```python
from build123d import *

# Parameters (mm, degrees)
SKETCH1_R                 = 20
BOSS_EXTRUDE1_DEPTH       = 25
BOSS_EXTRUDE2_START       = 100
SKETCH2_R                 = 20
BOSS_EXTRUDE2_DEPTH       = 100
BOSS_EXTRUDE4_START       = -100
SKETCH6_R                 = 20
BOSS_EXTRUDE4_DEPTH       = 100
SKETCH7_R                 = 25
CUT_EXTRUDE2_DEPTH        = 40
SKETCH8_R                 = 25
SKETCH8_R_2               = 22.5
BOSS_EXTRUDE7_DEPTH       = 40
SKETCH9_R                 = 25
BOSS_EXTRUDE8_DEPTH       = 2
BOSS_EXTRUDE10_DEPTH      = 38
CUT_EXTRUDE3_DEPTH        = 25
SKETCH12_R                = 25
CUT_EXTRUDE4_DEPTH        = 75
BOSS_EXTRUDE11_START      = 50
SKETCH14_R                = 20
BOSS_EXTRUDE11_DEPTH      = 50
BOSS_EXTRUDE12_DEPTH      = 10
BOSS_EXTRUDE12_DEPTH_BACK = 50
SKETCH13_R                = 37.5
SKETCH17_R                = 32.5
CUT_EXTRUDE5_DEPTH        = 50
BOSS_EXTRUDE13_START      = 2
SKETCH18_R                = 37.5
SKETCH18_R_2              = 32.5
BOSS_EXTRUDE13_DEPTH      = 2
SKETCH21_R                = 37.5
SKETCH21_R_2              = 32.5
CUT_EXTRUDE6_DEPTH        = 2
SKETCH22_R                = 1.5
CUT_EXTRUDE7_DEPTH        = 10
BOSS_EXTRUDE14_START      = 5
SKETCH27_R                = 32.5
BOSS_EXTRUDE14_DEPTH      = 5
CUT_EXTRUDE8_DEPTH        = 5
SKETCH29_R                = 1
CUT_EXTRUDE9_DEPTH        = 2.5
SKETCH30_R                = 1
CUT_EXTRUDE10_DEPTH       = 2.5


with BuildPart() as part:
    # Sketch1 → Boss-Extrude1 (new body)
    with BuildSketch(Plane(origin=(0, 0, 0), x_dir=(1, 0, 0), z_dir=(0, 1, 0))):
        with Locations(Location((0, 0, 0), (0, 0, 270))):
            Circle(SKETCH1_R)
        Polygon((14.43375673, 0), (7.216878365, 12.5), (-7.216878365, 12.5), (-14.43375673, 0), (-7.216878365, -12.5), (7.216878365, -12.5), align=None, mode=Mode.SUBTRACT)
    extrude(amount=BOSS_EXTRUDE1_DEPTH)

    # Sketch2 → Boss-Extrude2 (add)
    with BuildSketch(Plane.XZ.offset(BOSS_EXTRUDE2_START)):
        with Locations(Location((0, 0, 0), (0, 0, 270))):
            Circle(SKETCH2_R)
    extrude(amount=-BOSS_EXTRUDE2_DEPTH)

    # Sketch6 → Boss-Extrude4 (add)
    with BuildSketch(Plane(origin=(0, 25, 0), x_dir=(1, 0, 0), z_dir=(0, 1, 0)).offset(BOSS_EXTRUDE4_START)):
        with Locations(Location((0, 0, 0), (0, 0, 90))):
            Circle(SKETCH6_R)
    extrude(amount=BOSS_EXTRUDE4_DEPTH)

    # Sketch7 → Cut-Extrude2 (cut)
    with BuildSketch(Plane(origin=(20, 0, 0), x_dir=(0, 0, -1), z_dir=(1, 0, 0))):
        with Locations((0, 39.286563349)):
            Circle(SKETCH7_R)
    extrude(amount=-CUT_EXTRUDE2_DEPTH, mode=Mode.SUBTRACT)

    # Sketch8 → Boss-Extrude7 (add)
    with BuildSketch(Plane(origin=(20, 0, 0), x_dir=(0, 0, -1), z_dir=(1, 0, 0))):
        with Locations((0, 39.252781264)):
            Circle(SKETCH8_R)
        with Locations((0, 39.252781264)):
            Circle(SKETCH8_R_2, mode=Mode.SUBTRACT)
    extrude(amount=-BOSS_EXTRUDE7_DEPTH)

    # Sketch9 → Boss-Extrude8 (add)
    with BuildSketch(Plane(origin=(20, 0, 0), x_dir=(0, 0, -1), z_dir=(1, 0, 0))):
        with Locations((0, 39.252781264)):
            Circle(SKETCH9_R)
    extrude(amount=-BOSS_EXTRUDE8_DEPTH)

    # Sketch10 → Boss-Extrude10 (add)
    with BuildSketch(Plane.ZY.offset(-18)):
        with BuildLine():
            Line((-15.081099266, 22.555163323), (15.081099266, 22.555163323))
            ThreePointArc((15.081099266, 22.555163323), (0, 16.752781264), (-15.081099266, 22.555163323))
        make_face()
    extrude(amount=BOSS_EXTRUDE10_DEPTH)

    # Sketch11 → Cut-Extrude3 (cut)
    with BuildSketch(Plane.XZ.offset(100)):
        Polygon((12.5, 7.216878365), (0, 14.43375673), (0, 0), (12.5, 0), align=None)
        Polygon((0, 0), (0, 14.43375673), (-12.5, 7.216878365), (-12.5, -7.216878365), (0, -14.43375673), (12.5, -7.216878365), (12.5, 0), align=None)
    extrude(amount=-CUT_EXTRUDE3_DEPTH, mode=Mode.SUBTRACT)

    # Sketch12 → Cut-Extrude4 (cut)
    with BuildSketch(Plane(origin=(20, 0, 0), x_dir=(0, 0, -1), z_dir=(1, 0, 0))):
        with Locations((0, 39.252781264)):
            Circle(SKETCH12_R)
    extrude(amount=-CUT_EXTRUDE4_DEPTH, mode=Mode.SUBTRACT)

    # Sketch14 → Boss-Extrude11 (add)
    with BuildSketch(Plane.XZ.offset(100).offset(BOSS_EXTRUDE11_START)):
        with Locations(Location((0, 0, 0), (0, 0, 270))):
            Circle(SKETCH14_R)
        Polygon((0, -14.43375673), (12.5, -7.216878365), (12.5, 7.216878365), (0, 14.43375673), (-12.5, 7.216878365), (-12.5, -7.216878365), align=None, mode=Mode.SUBTRACT)
    extrude(amount=-BOSS_EXTRUDE11_DEPTH)

    # Sketch13 → Boss-Extrude12 (add, two sides: drawn at the far end of the back side and taken through both)
    with BuildSketch(Plane(origin=(20, 0, 0), x_dir=(0, 0, -1), z_dir=(1, 0, 0)).offset(-BOSS_EXTRUDE12_DEPTH_BACK)):
        with Locations((0, 39.33472939)):
            Circle(SKETCH13_R)
    extrude(amount=BOSS_EXTRUDE12_DEPTH + BOSS_EXTRUDE12_DEPTH_BACK)

    # Sketch17 → Cut-Extrude5 (cut)
    with BuildSketch(Plane(origin=(30, 0, 0), x_dir=(0, 0, -1), z_dir=(1, 0, 0))):
        with Locations((0, 39.33472939)):
            Circle(SKETCH17_R)
    extrude(amount=-CUT_EXTRUDE5_DEPTH, mode=Mode.SUBTRACT)

    # Sketch18 → Boss-Extrude13 (add)
    with BuildSketch(Plane(origin=(30, 0, 0), x_dir=(0, 0, -1), z_dir=(1, 0, 0)).offset(BOSS_EXTRUDE13_START)):
        with Locations((0, 39.33472939)):
            Circle(SKETCH18_R)
        with Locations((0, 39.33472939)):
            Circle(SKETCH18_R_2, mode=Mode.SUBTRACT)
    extrude(amount=-BOSS_EXTRUDE13_DEPTH)

    # Sketch21 → Cut-Extrude6 (cut)
    with BuildSketch(Plane(origin=(32, 0, 0), x_dir=(0, 0, -1), z_dir=(1, 0, 0))):
        with Locations((0, 39.33472939)):
            Circle(SKETCH21_R)
        with Locations((0, 39.33472939)):
            Circle(SKETCH21_R_2, mode=Mode.SUBTRACT)
    extrude(amount=-CUT_EXTRUDE6_DEPTH, mode=Mode.SUBTRACT)

    # Sketch22 → Cut-Extrude7 (cut)
    with BuildSketch(Plane(origin=(30, 0, 0), x_dir=(0, 0, -1), z_dir=(1, 0, 0))):
        with Locations((0, 74.33472939)):
            Circle(SKETCH22_R)
        with Locations((0, 4.33472939)):
            Circle(SKETCH22_R)
    extrude(amount=-CUT_EXTRUDE7_DEPTH, mode=Mode.SUBTRACT)

    # Sketch27 → Boss-Extrude14 (add)
    with BuildSketch(Plane(origin=(-20, 0, 0), x_dir=(0, 0, -1), z_dir=(1, 0, 0)).offset(BOSS_EXTRUDE14_START)):
        with Locations((0, 39.33472939)):
            Circle(SKETCH27_R)
    extrude(amount=-BOSS_EXTRUDE14_DEPTH)

    # Sketch28 → Cut-Extrude8 (cut)
    with BuildSketch(Plane(origin=(-15, 0, 0), x_dir=(0, 0, -1), z_dir=(1, 0, 0))):
        with BuildLine():
            ThreePointArc((-6.975, 64.469273085), (-7.975, 65.469273085), (-8.975, 64.469273085))
            Line((-8.975, 64.469273085), (-6.975, 64.469273085))
        make_face()
        with BuildLine():
            Line((-6.975, 64.469273085), (-8.975, 64.469273085))
            ThreePointArc((-8.975, 64.469273085), (-7.975, 63.469273085), (-6.975, 64.469273085))
        make_face()
        with BuildLine():
            ThreePointArc((8.975, 64.469273085), (7.975, 65.469273085), (6.975, 64.469273085))
            Line((6.975, 64.469273085), (8.975, 64.469273085))
        make_face()
        with BuildLine():
            Line((8.975, 64.469273085), (6.975, 64.469273085))
            ThreePointArc((6.975, 64.469273085), (7.975, 63.469273085), (8.975, 64.469273085))
        make_face()
    extrude(amount=-CUT_EXTRUDE8_DEPTH, mode=Mode.SUBTRACT)

    # Sketch29 → Cut-Extrude9 (cut)
    with BuildSketch(Plane(origin=(-20, 0, 0), x_dir=(0, 0, -1), z_dir=(1, 0, 0))):
        with Locations((7.975, 64.469273085)):
            Circle(SKETCH29_R)
    extrude(amount=-CUT_EXTRUDE9_DEPTH, mode=Mode.SUBTRACT)

    # Sketch30 → Cut-Extrude10 (cut)
    with BuildSketch(Plane(origin=(-20, 0, 0), x_dir=(0, 0, -1), z_dir=(1, 0, 0))):
        with Locations((-7.975, 64.469273085)):
            Circle(SKETCH30_R)
    extrude(amount=-CUT_EXTRUDE10_DEPTH, mode=Mode.SUBTRACT)


solid = part.part
```
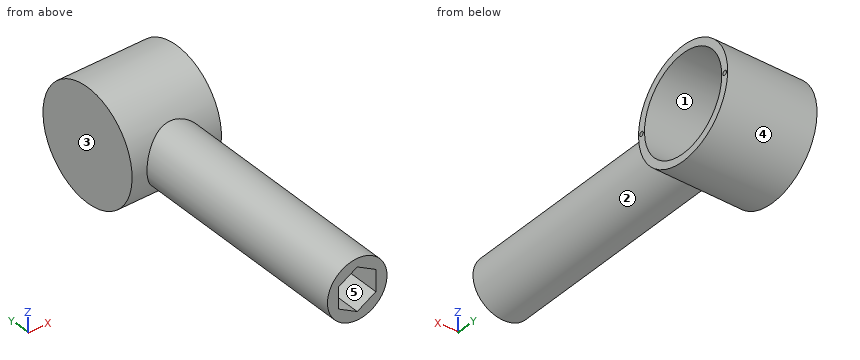
Build history of the part. All positions in model axes, mm. Face numbers are marked on the shaded views. A direction names the side the tool comes from. Round coordinates to 2 decimals unless told otherwise and drop trailing zeros. Order: outer loops, then holes, each group sorted by start corner. A loop starts at its lowest first (then second) coordinate and runs counter-clockwise, first axis right, second up. Notation, with made-up numbers: (20, 50.5) - (71, 50.5) arc R20 ccw to (71, 77.5) - close; hole circle Ø1 at (76, -15). An arc over 180 degrees is marked (long way). Use a Markdown table: item, result.
1) Pull direction Z, two halves, no side cores. Call the marked faces 3, 4 and 5: pulls with the +Z half, pulls with the -Z half, needs draft (parallel to the pull), parting line crosses it, or undercut.
Recorded:
| item | result |
|---|---|
| face 3 | needs draft |
| face 4 | parting line crosses it |
| face 5 | undercut |
2) Saw through at B-B on x = -4.5. Write the cut outline in (y, z), and give its area (3 significant figures).
Recorded:
| item | result |
|---|---|
| outline | (-150, -19.49) - (7.3, -19.49) arc R37.5 ccw (long way) to (7.3, 19.49) - (-150, 19.49) - (-150, 11.84) - (-75, 11.84) - (-75, -11.84) - (-150, -11.84) - close; hole circle Ø65 at (39.33, 0) |
| area | 5,310 mm² |
3) Saw through at C-C on y = -65.5. Write the cut outline in (x, z), and give its area (3 significant figures).
Recorded:
| item | result |
|---|---|
| outline | circle Ø40 at (0, 0) |
| area | 1,260 mm² |
4) Wall check: L1, parallel to Y at x = 26.25, z = 0; L2, parallel to Y at x = 5, z = 0; L3, parallel to X at y = 45, z = -23. Give the ranges that are in metal, low to high.
Recorded:
| item | result |
|---|---|
| L1 | y = 1.83 to 2.83, 5.83 to 6.83, 71.83 to 72.83, 75.83 to 76.83 |
| L2 | y = -75 to 6.83, 71.83 to 76.83 |
| L3 | x = -30 to -15 |
5) Flat gauge pins, fed straight in: pin 1 Ø2 at (x, z) = (-9.5, 7.5) entering from +Y; pin 2 Ø3 at (y, z) = (-83.5, -14.5) entering from -X; pin 3 Ø4.5 at (y, z) = (-117.5, -1) entering from +X; pin 4 Ø1 at (x, y) = (-21.5, -21.5) entering from -Z. Where does each tip first touch, or does it go through?
Recorded:
| item | result |
|---|---|
| pin 1 | stops at y = 76.27 |
| pin 2 | stops at x = -15.2 |
| pin 3 | stops at x = 20 |
| pin 4 | passes through |
6) Tool access for the marked faces 1 and 2: list every direction of +Z, -Z, +X, -X, +Y, -Y with a clear straight run to the whole face (end or side of a thin tool).
Recorded:
| item | result |
|---|---|
| face 1 | +X |
| face 2 | -Y |
7) Saw through at A-A on y = -128.5. Write the cut outline in (x, z), and give its area (3 significant figures).
Recorded:
| item | result |
|---|---|
| outline | circle Ø40 at (0, 0); hole (-12.5, -7.22) - (0, -14.43) - (12.5, -7.22) - (12.5, 7.22) - (0, 14.43) - (-12.5, 7.22) - close |
| area | 715 mm² |
8) Saw through at D-D on z = 22. Write the cut outline in (x, y).
Recorded:
| item | result |
|---|---|
| outline | (-30, 8.97) - (30, 8.97) - (30, 15.41) - (-15, 15.41) - (-15, 63.26) - (30, 63.26) - (30, 69.7) - (-30, 69.7) - close |
